For this review, take the finished solid that the model builds, in its own axes (mm). A direction names the side the tool comes from. Give positions to 0.01 mm unless a question says otherwise; leave off trailing zeros. Loops run counter-clockwise (first coordinate to the right, second up) from the corner with the lowest first, then second, coordinate; pieces in that order, holes last.
```python
from build123d import *

# Parameters (mm, degrees)
SKETCH_1_R          = 1.5
SKETCH_1_R_2        = 1
EXTRUDE_1_DEPTH     = 2
CUT_EXTRUDE_START   = -10
CUT_EXTRUDE_1_DEPTH = 10
EXTRUDE_START       = -2
EXTRUDE_2_DEPTH     = 2


with BuildPart() as part:
    # Sketch 1 → Extrude 1 (new body)
    with BuildSketch(Plane(origin=(0, 0, 0), x_dir=(1, 0, 0), z_dir=(0, 1, 0))):
        with BuildLine():
            Line((-35, 15.5), (35, 15.5))
            ThreePointArc((35, 15.5), (36.414213562, 14.914213562), (37, 13.5))
            Line((37, 13.5), (37, -13.5))
            ThreePointArc((37, -13.5), (36.414213562, -14.914213562), (35, -15.5))
            Line((35, -15.5), (-35, -15.5))
            ThreePointArc((-35, -15.5), (-36.414213562, -14.914213562), (-37, -13.5))
            Line((-37, -13.5), (-37, 13.5))
            ThreePointArc((-37, 13.5), (-36.414213562, 14.914213562), (-35, 15.5))
        make_face()
        with Locations(Location((-34, 12.5, 0), (0, 0, 270))):
            Circle(SKETCH_1_R, mode=Mode.SUBTRACT)
        with Locations(Location((-34, -12.5, 0), (0, 0, 270))):
            Circle(SKETCH_1_R, mode=Mode.SUBTRACT)
        with Locations(Location((34, 12.5, 0), (0, 0, 270))):
            Circle(SKETCH_1_R, mode=Mode.SUBTRACT)
        with Locations(Location((34, -12.5, 0), (0, 0, 270))):
            Circle(SKETCH_1_R, mode=Mode.SUBTRACT)
        with Locations(Location((0, 11, 0), (0, 0, 270))):
            Circle(SKETCH_1_R_2, mode=Mode.SUBTRACT)
        with Locations(Location((-11, 0, 0), (0, 0, 270))):
            Circle(SKETCH_1_R_2, mode=Mode.SUBTRACT)
        with Locations(Location((0, -11, 0), (0, 0, 90))):
            Circle(SKETCH_1_R_2, mode=Mode.SUBTRACT)
        with Locations(Location((11, 0, 0), (0, 0, 90))):
            Circle(SKETCH_1_R_2, mode=Mode.SUBTRACT)
    extrude(amount=EXTRUDE_1_DEPTH)

    # Sketch 2 → Cut-Extrude 1 (cut)
    with BuildSketch(Plane(origin=(0, 2, 0), x_dir=(1, 0, 0), z_dir=(0, 1, 0)).offset(CUT_EXTRUDE_START)):
        with BuildLine():
            ThreePointArc((31.129544421, 13.372057779), (32.21340734, 14.909997234), (34, 15.5))
            Line((34, 15.5), (-34.000000062, 15.5))
            ThreePointArc((-34.000000062, 15.5), (-32.213407365, 14.909997253), (-31.129544421, 13.372057779))
            ThreePointArc((-31.129544421, 13.372057779), (-29.192502027, 8.274752588), (-26.580191252, 3.488262657))
            ThreePointArc((-26.580191252, 3.488262657), (-14.374020851, 11.15529545), (-0.242721863, 13.997895774))
            ThreePointArc((-0.242721863, 13.997895774), (0, 14), (0.242721863, 13.997895774))
            ThreePointArc((0.242721863, 13.997895774), (14.374020851, 11.15529545), (26.580191252, 3.488262657))
            ThreePointArc((26.580191252, 3.488262657), (29.192502027, 8.274752588), (31.129544421, 13.372057779))
        make_face()
        with BuildLine():
            ThreePointArc((37, 13.5), (36.414213562, 14.914213562), (35, 15.5))
            Line((35, 15.5), (34, 15.5))
            ThreePointArc((34, 15.5), (36.121320344, 14.621320344), (37, 12.5))
            Line((37, 12.5), (37, 13.5))
        make_face()
        with BuildLine():
            Line((37, -12.5), (37, 12.5))
            ThreePointArc((37, 12.5), (36.947873541, 11.943186219), (36.793305609, 11.405722258))
            ThreePointArc((36.793305609, 11.405722258), (33.849039363, 5.416414449), (29.949941227, 0))
            ThreePointArc((29.949941227, 0), (33.849039363, -5.416414449), (36.793305609, -11.405722258))
            ThreePointArc((36.793305609, -11.405722258), (36.947873541, -11.943186219), (37, -12.5))
        make_face()
        with BuildLine():
            ThreePointArc((24.082197813, 0), (15.011406824, 8.30476234), (3.846336647, 13.461266449))
            ThreePointArc((3.846336647, 13.461266449), (11.176956497, 8.430637193), (14, 0))
            ThreePointArc((14, 0), (11.176956497, -8.430637193), (3.846336647, -13.461266449))
            ThreePointArc((3.846336647, -13.461266449), (15.011406824, -8.30476234), (24.082197813, 0))
        make_face()
        with BuildLine():
            ThreePointArc((-36.793305609, 11.405722258), (-36.947873541, 11.943186219), (-37, 12.5))
            Line((-37, 12.5), (-37, -12.5))
            ThreePointArc((-37, -12.5), (-36.947873541, -11.943186219), (-36.793305609, -11.405722258))
            ThreePointArc((-36.793305609, -11.405722258), (-33.849039363, -5.416414449), (-29.949941227, 0))
            ThreePointArc((-29.949941227, 0), (-33.849039363, 5.416414449), (-36.793305609, 11.405722258))
        make_face()
        with BuildLine():
            Line((-34, -15.5), (34, -15.5))
            ThreePointArc((34, -15.5), (32.21340734, -14.909997234), (31.129544421, -13.372057779))
            ThreePointArc((31.129544421, -13.372057779), (29.192502027, -8.274752588), (26.580191252, -3.488262657))
            ThreePointArc((26.580191252, -3.488262657), (14.374020851, -11.15529545), (0.242721863, -13.997895774))
            ThreePointArc((0.242721863, -13.997895774), (0, -14), (-0.242721863, -13.997895774))
            ThreePointArc((-0.242721863, -13.997895774), (-14.374020851, -11.15529545), (-26.580191252, -3.488262657))
            ThreePointArc((-26.580191252, -3.488262657), (-29.192502027, -8.274752588), (-31.129544421, -13.372057779))
            ThreePointArc((-31.129544421, -13.372057779), (-32.21340734, -14.909997234), (-34, -15.5))
        make_face()
        with BuildLine():
            Line((37, -13.5), (37, -12.5))
            ThreePointArc((37, -12.5), (36.121320344, -14.621320344), (34, -15.5))
            Line((34, -15.5), (35, -15.5))
            ThreePointArc((35, -15.5), (36.414213562, -14.914213562), (37, -13.5))
        make_face()
        with BuildLine():
            ThreePointArc((-34, -15.5), (-36.121320344, -14.621320344), (-37, -12.5))
            Line((-37, -12.5), (-37, -13.5))
            ThreePointArc((-37, -13.5), (-36.414213562, -14.914213562), (-35, -15.5))
            Line((-35, -15.5), (-34, -15.5))
        make_face()
        with BuildLine():
            ThreePointArc((-37, 12.5), (-36.121320365, 14.621320322), (-34.000000062, 15.5))
            Line((-34.000000062, 15.5), (-35, 15.5))
            ThreePointArc((-35, 15.5), (-36.414213562, 14.914213562), (-37, 13.5))
            Line((-37, 13.5), (-37, 12.5))
        make_face()
        with BuildLine():
            ThreePointArc((-3.846336647, -13.461266449), (-14, 0), (-3.846336647, 13.461266449))
            ThreePointArc((-3.846336647, 13.461266449), (-15.011406824, 8.30476234), (-24.082197813, 0))
            ThreePointArc((-24.082197813, 0), (-15.011406824, -8.30476234), (-3.846336647, -13.461266449))
        make_face()
    extrude(amount=CUT_EXTRUDE_1_DEPTH, mode=Mode.SUBTRACT)

    # Sketch 3 → Extrude 2 (add)
    with BuildSketch(Plane(origin=(0, 2, 0), x_dir=(1, 0, 0), z_dir=(0, 1, 0)).offset(EXTRUDE_START)):
        with BuildLine():
            Line((-10.083439521, 11.100962324), (-9.356776872, 10.413967859))
            ThreePointArc((-9.356776872, 10.413967859), (-6.775105817, 12.251446493), (-3.846336647, 13.461266449))
            ThreePointArc((-3.846336647, 13.461266449), (-7.014162346, 12.411321608), (-10.083439521, 11.100962324))
        make_face()
        with BuildLine():
            Line((10.083439521, 11.100962324), (9.356776872, 10.413967859))
            ThreePointArc((9.356776872, 10.413967859), (6.775105817, 12.251446493), (3.846336647, 13.461266449))
            ThreePointArc((3.846336647, 13.461266449), (7.014162346, 12.411321608), (10.083439521, 11.100962324))
        make_face()
        with BuildLine():
            Line((-10.083439521, -11.100962324), (-9.356776872, -10.413967859))
            ThreePointArc((-9.356776872, -10.413967859), (-6.775105817, -12.251446493), (-3.846336647, -13.461266449))
            ThreePointArc((-3.846336647, -13.461266449), (-7.014162346, -12.411321608), (-10.083439521, -11.100962324))
        make_face()
        with BuildLine():
            Line((10.083439521, -11.100962324), (9.356776872, -10.413967859))
            ThreePointArc((9.356776872, -10.413967859), (6.775105817, -12.251446493), (3.846336647, -13.461266449))
            ThreePointArc((3.846336647, -13.461266449), (7.014162346, -12.411321608), (10.083439521, -11.100962324))
        make_face()
    extrude(amount=EXTRUDE_2_DEPTH)


solid = part.part
```
Q1. Consider section B-B on x = 11. Give the boundary of the cut face in (y, z), plus the area to 3 significant figures.
Answers:
outline: (0, -12.33) - (2, -12.33) - (2, -10.65) - (0, -10.65) - close; (0, -8.66) - (2, -8.66) - (2, -1) - (0, -1) - close; (0, 1) - (2, 1) - (2, 8.66) - (0, 8.66) - close; (0, 10.65) - (2, 10.65) - (2, 12.33) - (0, 12.33) - close
area: 37.4 mm2
Q2. Consider section D-D on z = -5.5. Give the boundary of the cut face in (x, y), plus the area to 3 significant figures.
Answers:
outline: (-33.9, 0) - (-27.78, 0) - (-27.78, 2) - (-33.9, 2) - close; (-24.21, 0) - (-18.74, 0) - (-18.74, 2) - (-24.21, 2) - close; (-12.87, 0) - (12.87, 0) - (12.87, 2) - (-12.87, 2) - close; (18.74, 0) - (24.21, 0) - (24.21, 2) - (18.74, 2) - close; (27.78, 0) - (33.9, 0) - (33.9, 2) - (27.78, 2) - close
area: 97.8 mm2
Q3. For pin 1 Ø1.8 at (x, z) = (34, -12.5) entering from -Y; pin 2 Ø4 at (x, z) = (4.5, 9.5) entering from -Y, all flat-tipped, find the tip position at first contact; note any pin that passes through.
Answers:
pin 1: passes through
pin 2: stops at y = 0
Q4. Consider section A-A on z = 2. Give the boundary of the cut face in (x, y).
Answers:
outline: (-31.55, 0) - (-22.37, 0) - (-22.37, 2) - (-31.55, 2) - close; (-13.86, 0) - (13.86, 0) - (13.86, 2) - (-13.86, 2) - close; (22.37, 0) - (31.55, 0) - (31.55, 2) - (22.37, 2) - close
Q5. For probe 1 along Z at (x, y) = (-33, 1.05); probe 2 along X at (y, z) = (1.2, 6.5); probe 3 along X at (y, z) = (0.2, 2), list the stretches that pass through material, from the lowest coordinate up.
Answers:
probe 1: z = -15.33 to -13.62, -11.38 to -4.06, 4.06 to 11.38, 13.62 to 15.33
probe 2: x = -34.48 to -28.32, -22.87 to -17.51, -12.4 to 12.4, 17.51 to 22.87, 28.32 to 34.48
probe 3: x = -31.55 to -22.37, -13.86 to 13.86, 22.37 to 31.55
Q6. Mouldability with a two-part tool opening along X and no side actions: class faces 6 (the flat face through (-1, 0, 0)), 7 (the cylindrical face through (-10, 1, 0)), 8 (the cylindrical face through (-33.801, 0.986, -5.336)) as +X half, -X half, draft (parallel to the pull), parting line (faces both ways), or undercut.
Answers:
face 6: draft
face 7: undercut
face 8: -X half
Q7. Consider section C-C on x = -22. Give the boundary of the cut face in (y, z).
Answers:
outline: (0, -7.11) - (2, -7.11) - (2, -2.4) - (0, -2.4) - close; (0, 2.4) - (2, 2.4) - (2, 7.11) - (0, 7.11) - close
Q8. Machinability: for faces 1 (the cylindrical face through (-29.16, 0.986, 8.205)), 2 (the flat face through (-1, 2, 0)), 3 (the cylindrical face through (-33.9, 1, 5.5)), 4 (the cylindrical face through (-14, 1, 0)), 5 (the cylindrical face through (-29.224, 0.986, -8.344)), which of the approach directions +Z, -Z, +X, -X, +Y, -Y give a long, thin tool a straight path to every point of the face, cutting with its end or side? Answer none if there is none.
Answers:
face 1: +Z, +Y, -Y
face 2: +Z, -Z, +X, -X, +Y
face 3: -X, +Y, -Y
face 4: +Y, -Y
face 5: -Z, +Y, -Y
